Geometry: final body of the model. Coordinates: model frame, mm. A direction names the side the tool comes from. Give positions to 0.01 mm unless a question says otherwise; leave off trailing zeros. Loops run counter-clockwise (first coordinate to the right, second up) from the corner with the lowest first, then second, coordinate; pieces in that order, holes last.
1. First-contact query: P1, Ø1.4, axis at x = 63.5, z = 3, coming from the -Y side; P2, Ø1.1, axis at x = 71.5, z = 4.5, coming from the -Y side; P3, Ø3, axis at y = 36.5, z = 3, coming from the +X side; P4, Ø2, axis at x = 76.17, y = 8.42, coming from the +Z side. Flat tips, straight axial feed; report the tip coordinate or a pass-through.
2. Section A-A, the plane y = 15. Output: boundary loops of the cut face in (x, z).
3. Section D-D, the plane z = 8. State how many separate pieces and enclosed holes the cut face has, then the cut area to 3 significant figures.
4. Access query for faces 5 (the face through (71.515, 21.67, 6.958)), 6 (the face through (8, 45.25, 5)), 7 (the face through (18.611, 28, 2)). Directions: +Z, -Z, +X, -X, +Y, -Y. A direction counts if a zero-diameter tool reaches every point of the face in a straight line with its end or side. Return the directions, or none.
5. Section C-C, the plane x = 15.5. Output: boundary loops of the cut face in (y, z).
6. Material intervals for line 1 along Y through (x, z) = (76, 8.5); line 2 along X through (y, z) = (28.5, 2); line 3 along Y through (x, z) = (38.5, 2.25), sorted ascending.
7. Section B-B, the plane x = 67.5. Output: boundary loops of the cut face in (y, z), then the cut area to 3 significant figures.
8. Draft query along Y for faces 1 (the face through (75, 55, 0)), 2 (the face through (25, 30.686, 2)), 3 (the face through (8, 34.334, 5)), 4 (the face through (31, 23.353, 7)). Return one class per face: +Y half, -Y half, draft (parallel to the pull), parting line (faces both ways), or undercut.
from build123d import *

# Parameters (mm, degrees)
SKETCH_1_W           = 85
SKETCH_1_H           = 65
EXTRUDE_1_DEPTH      = 10
CUT_EXTRUDE_1_REACH  = 109.471
SKETCH_2_R           = 1.7
CUT_EXTRUDE_2_REACH  = 109.471
SKETCH_3_W           = 85
SKETCH_3_H           = 65
CUT_EXTRUDE_4_REACH  = 102.464
CUT_EXTRUDE_7_DEPTH  = 6
CUT_EXTRUDE_8_DEPTH  = 6
CUT_EXTRUDE_11_DEPTH = 4
SKETCH_8_W           = 8
SKETCH_8_H           = 5
CUT_EXTRUDE_12_DEPTH = 1
SKETCH_10_W          = 5.4
SKETCH_10_H          = 6
SKETCH_10_W_2        = 4
EXTRUDE_2_DEPTH      = 3.04
SKETCH_11_W          = 4.2
SKETCH_11_H          = 5
EXTRUDE_3_DEPTH      = 2.300115
SKETCH_12_W          = 12
SKETCH_12_H          = 6
EXTRUDE_4_DEPTH      = 2.89
SKETCH_13_W          = 6.499986347
SKETCH_13_H          = 5.115524378
EXTRUDE_5_DEPTH      = 3.6
SKETCH_14_W          = 6
SKETCH_14_H          = 7
EXTRUDE_6_DEPTH      = 2.890002
SKETCH_15_W          = 14
SKETCH_15_H          = 4.4
CUT_EXTRUDE_13_DEPTH = 6
CHAMFER_1_SIZE       = 1
CHAMFER_2_SIZE       = 0.6
CHAMFER_3_SIZE       = 0.6
CHAMFER_4_SIZE       = 0.6
CHAMFER_5_SIZE       = 0.6
CHAMFER_6_SIZE       = 0.6


with BuildPart() as part:
    # 草图1 → 凸台-拉伸1 (new body)
    with BuildSketch(Plane.XY):
        with Locations((42.5, 32.5)):
            Rectangle(SKETCH_1_W, SKETCH_1_H)
    extrude(amount=EXTRUDE_1_DEPTH)

    # 草图2 → 切除-拉伸1 (cut, up to next)
    with BuildSketch(Plane(origin=(0, 0, 0), x_dir=(-1, 0, 0), z_dir=(0, 0, -1)), mode=Mode.PRIVATE) as cut_extrude_1_sk1:
        with Locations((-76.166921514, 56.442524765)):
            Circle(SKETCH_2_R)
    cut_extrude_1_tool1 = extrude(cut_extrude_1_sk1.sketch, amount=-CUT_EXTRUDE_1_REACH, mode=Mode.PRIVATE) & part.part
    # 草图2 → 切除-拉伸1 (cut, up to next)
    with BuildSketch(Plane(origin=(0, 0, 0), x_dir=(-1, 0, 0), z_dir=(0, 0, -1)), mode=Mode.PRIVATE) as cut_extrude_1_sk2:
        with Locations((-8.888803658, 56.442524765)):
            Circle(SKETCH_2_R)
    cut_extrude_1_tool2 = extrude(cut_extrude_1_sk2.sketch, amount=-CUT_EXTRUDE_1_REACH, mode=Mode.PRIVATE) & part.part
    # 草图2 → 切除-拉伸1 (cut, up to next)
    with BuildSketch(Plane(origin=(0, 0, 0), x_dir=(-1, 0, 0), z_dir=(0, 0, -1)), mode=Mode.PRIVATE) as cut_extrude_1_sk3:
        with Locations((-76.166921514, 8.41508509)):
            Circle(SKETCH_2_R)
    cut_extrude_1_tool3 = extrude(cut_extrude_1_sk3.sketch, amount=-CUT_EXTRUDE_1_REACH, mode=Mode.PRIVATE) & part.part
    # 草图2 → 切除-拉伸1 (cut, up to next)
    with BuildSketch(Plane(origin=(0, 0, 0), x_dir=(-1, 0, 0), z_dir=(0, 0, -1)), mode=Mode.PRIVATE) as cut_extrude_1_sk4:
        with Locations((-8.888803658, 8.41508509)):
            Circle(SKETCH_2_R)
    cut_extrude_1_tool4 = extrude(cut_extrude_1_sk4.sketch, amount=-CUT_EXTRUDE_1_REACH, mode=Mode.PRIVATE) & part.part
    add(cut_extrude_1_tool1.solids().sort_by_distance((76.166922, 56.442525, 0))[0], mode=Mode.SUBTRACT)
    add(cut_extrude_1_tool2.solids().sort_by_distance((8.888804, 56.442525, 0))[0], mode=Mode.SUBTRACT)
    add(cut_extrude_1_tool3.solids().sort_by_distance((76.166922, 8.415085, 0))[0], mode=Mode.SUBTRACT)
    add(cut_extrude_1_tool4.solids().sort_by_distance((8.888804, 8.415085, 0))[0], mode=Mode.SUBTRACT)

    # 草图3 → 切除-拉伸2 (cut, up to next)
    with BuildSketch(Plane(origin=(0, 0, 0), x_dir=(-1, 0, 0), z_dir=(0, 0, -1)), mode=Mode.PRIVATE) as cut_extrude_2_sk1:
        with Locations((-42.5, 32.5)):
            Rectangle(SKETCH_3_W, SKETCH_3_H)
        Polygon((-5, 33.462892894), (-5.871324699, 34.334217592), (-5.87504445, 53.137061214), (-5, 54.017366187), (-5, 57.982143592), (-6.992565577, 59.974709169), (-23.773560915, 59.974709169), (-24.394872914, 59.353397171), (-54.61482093, 59.349677419), (-55.245113202, 59.974709169), (-77.982184232, 59.974709169), (-79.974749809, 57.982143592), (-79.97474981, 54.295829484), (-78.032030648, 52.353110322), (-78.028310897, 12.45999492), (-79.97474981, 10.508295484), (-79.97474981, 6.992565577), (-77.982184232, 5), (-74.414239441, 5), (-73.152434681, 6.26180476), (-60.043505207, 6.265524511), (-58.772720173, 5), (-32.926479725, 5), (-31.743585303, 6.182894422), (-17.461559563, 6.186614173), (-16.269684867, 5), (-6.992565577, 5), (-5, 6.992565577), align=None, mode=Mode.SUBTRACT)
    cut_extrude_2_tool1 = extrude(cut_extrude_2_sk1.sketch, amount=-CUT_EXTRUDE_2_REACH, mode=Mode.PRIVATE) & part.part
    add(cut_extrude_2_tool1.solids().sort_by_distance((42.5, 63.929953, 0))[0], mode=Mode.SUBTRACT)

    # 草图4 → 切除-拉伸4 (cut, up to next)
    with BuildSketch(Plane(origin=(0, 0, 0), x_dir=(-1, 0, 0), z_dir=(0, 0, -1)), mode=Mode.PRIVATE) as cut_extrude_4_sk1:
        Polygon((-73.152434681, 6.26180476), (-73.152434681, 20.032317315), (-69.831576581, 23.353175415), (-46.787984184, 23.353175415), (-20.851296271, 23.353175415), (-17.461559563, 19.963438707), (-17.461559563, 6.186614173), (-17.461559563, 0.193960815), (-73.152434681, 0.193960815), align=None)
    cut_extrude_4_tool1 = extrude(cut_extrude_4_sk1.sketch, amount=-CUT_EXTRUDE_4_REACH, mode=Mode.PRIVATE) & part.part
    add(cut_extrude_4_tool1.solids().sort_by_distance((45.311727, 11.681443, 0))[0], mode=Mode.SUBTRACT)

    # 草图5 → 切除-拉伸7 (cut)
    with BuildSketch(Plane(origin=(0, 0, 0), x_dir=(-1, 0, 0), z_dir=(0, 0, -1))):
        Polygon((-24.394872914, 59.353397171), (-24.394872914, 53.906418167), (-25.526104495, 52.774908066), (-53.482640788, 52.774908066), (-54.614150889, 53.906139647), (-54.61482093, 59.349677419), align=None)
    extrude(amount=-CUT_EXTRUDE_7_DEPTH, mode=Mode.SUBTRACT)

    # 草图6 → 切除-拉伸8 (cut)
    with BuildSketch(Plane(origin=(0, 0, 0), x_dir=(-1, 0, 0), z_dir=(0, 0, -1))):
        Polygon((-5.871324699, 34.334217592), (-11.136213102, 34.334217592), (-11.687697798, 35.836171197), (-11.687697798, 43.836171197), (-10.273484235, 45.250384759), (-5.873484235, 45.250384759), align=None)
    extrude(amount=-CUT_EXTRUDE_8_DEPTH, mode=Mode.SUBTRACT)

    # 草图7 → 切除-拉伸11 (cut)
    with BuildSketch(Plane(origin=(0, 0, 0), x_dir=(-1, 0, 0), z_dir=(0, 0, -1))):
        Polygon((-74.432117646, 51.26230094), (-76.432117646, 51.26230094), (-78.031928938, 51.26230094), (-78.029847328, 28.93771831), (-75.029847328, 28.93771831), (-75.029847328, 13.93771831), (-73.152434681, 12.060305663), (-73.152434681, 20.032317315), (-69.831576581, 23.353175415), (-20.851296271, 23.353175415), (-17.461559563, 19.963438707), (-17.461559563, 6.186614173), (-16.269684867, 5), (-12.014024847, 5), (-12.014024847, 10.599811284), (-10.599811284, 12.014024847), (-6.599811284, 12.014024847), (-5, 12.014024847), (-5, 33.462892894), (-5.871324699, 34.334217592), (-11.136213102, 34.334217592), (-11.687697798, 35.836171197), (-11.687697798, 43.836171197), (-10.273484235, 45.250384759), (-5.873484235, 45.250384759), (-5.87504445, 53.137061214), (-9.87504445, 53.137061214), (-12.071959353, 55.333976117), (-12.071959353, 58.333976117), (-23.061659554, 58.333976117), (-23.732127818, 57.663342778), (-24.394872914, 57.663261201), (-24.394872914, 53.906418167), (-25.526104495, 52.774908066), (-53.482640788, 52.774908066), (-54.614150889, 53.906139647), (-54.61482093, 59.349677419), (-55.245113202, 59.974709169), (-71.319520701, 59.974709169), (-71.319520701, 58.374897885), (-71.319520701, 54.374897885), align=None)
    extrude(amount=-CUT_EXTRUDE_11_DEPTH, mode=Mode.SUBTRACT)

    # 草图8 → 切除-拉伸12 (cut)
    with BuildSketch(Plane(origin=(0, 0, 4), x_dir=(-1, 0, 0), z_dir=(0, 0, -1))):
        with Locations((-69.348077333, 43.45871309)):
            Rectangle(SKETCH_8_W, SKETCH_8_H)
    extrude(amount=-CUT_EXTRUDE_12_DEPTH, mode=Mode.SUBTRACT)

    # 草图10 → 凸台-拉伸2 (add)
    with BuildSketch(Plane(origin=(0, 0, 4), x_dir=(-1, 0, 0), z_dir=(0, 0, -1))):
        with Locations((-44.246532103, 31.889800214)):
            Rectangle(SKETCH_10_W, SKETCH_10_H)
        with Locations((-39.546532103, 31.889800214)):
            Rectangle(SKETCH_10_W_2, SKETCH_10_H)
        with Locations((-34.846532103, 31.889800214)):
            Rectangle(SKETCH_10_W, SKETCH_10_H)
    extrude(amount=EXTRUDE_2_DEPTH)

    # 草图11 → 凸台-拉伸3 (add)
    with BuildSketch(Plane(origin=(0, 0, 4), x_dir=(-1, 0, 0), z_dir=(0, 0, -1))):
        with Locations((-38.731800654, 41.192864876)):
            Rectangle(SKETCH_11_W, SKETCH_11_H)
    extrude(amount=EXTRUDE_3_DEPTH)

    # 草图12 → 凸台-拉伸4 (add)
    with BuildSketch(Plane(origin=(0, 0, 4), x_dir=(-1, 0, 0), z_dir=(0, 0, -1))):
        with Locations((-24.610605003, 27.685920752)):
            Rectangle(SKETCH_12_W, SKETCH_12_H)
    extrude(amount=EXTRUDE_4_DEPTH)

    # 草图13 → 凸台-拉伸5 (add)
    with BuildSketch(Plane(origin=(0, 0, 4), x_dir=(-1, 0, 0), z_dir=(0, 0, -1))):
        with Locations((-61.319842519, 38.061085021)):
            Rectangle(SKETCH_13_W, SKETCH_13_H)
    extrude(amount=EXTRUDE_5_DEPTH)

    # 草图14 → 凸台-拉伸6 (add)
    with BuildSketch(Plane(origin=(0, 0, 4), x_dir=(-1, 0, 0), z_dir=(0, 0, -1))):
        with Locations((-62.740849727, 27.111901224)):
            Rectangle(SKETCH_14_W, SKETCH_14_H)
    extrude(amount=EXTRUDE_6_DEPTH)

    # 草图15 → 切除-拉伸13 (cut)
    with BuildSketch(Plane.XY.offset(10)):
        with Locations((48.428848604, 25.553175415)):
            Rectangle(SKETCH_15_W, SKETCH_15_H)
    extrude(amount=-CUT_EXTRUDE_13_DEPTH, mode=Mode.SUBTRACT)

    # 倒角1
    chamfer_1_edges = [part.edges().sort_by_distance(p)[0] for p in [
        (55.428848604, 23.353175415, 7),
        (55.428848604, 27.753175415, 7),
        (41.428848604, 27.753175415, 7),
        (41.428848604, 23.353175415, 7),
    ]]
    chamfer(chamfer_1_edges, length=CHAMFER_1_SIZE)

    # 倒角2
    chamfer_2_edges = [part.edges().sort_by_distance(p)[0] for p in [
        (64.569835693, 38.061085021, 4),
        (61.31984252, 35.503322832, 4),
        (58.069849346, 38.061085021, 4),
        (61.31984252, 40.61884721, 4),
    ]]
    chamfer(chamfer_2_edges, length=CHAMFER_2_SIZE)

    # 倒角3
    chamfer_3_edges = [part.edges().sort_by_distance(p)[0] for p in [
        (39.546532103, 28.889800214, 4),
        (46.946532103, 31.889800214, 4),
        (39.546532103, 34.889800214, 4),
        (32.146532103, 31.889800214, 4),
    ]]
    chamfer(chamfer_3_edges, length=CHAMFER_3_SIZE)

    # 倒角4
    chamfer_4_edges = [part.edges().sort_by_distance(p)[0] for p in [
        (30.610605003, 27.685920752, 4),
        (24.610605003, 24.685920752, 4),
        (18.610605003, 27.685920752, 4),
        (24.610605003, 30.685920752, 4),
    ]]
    chamfer(chamfer_4_edges, length=CHAMFER_4_SIZE)

    # 倒角5
    chamfer_5_edges = [part.edges().sort_by_distance(p)[0] for p in [
        (40.831800654, 41.192864876, 4),
        (38.731800654, 38.692864876, 4),
        (36.631800654, 41.192864876, 4),
        (38.731800654, 43.692864876, 4),
    ]]
    chamfer(chamfer_5_edges, length=CHAMFER_5_SIZE)

    # 倒角6
    chamfer_6_edges = [part.edges().sort_by_distance(p)[0] for p in [
        (65.740849727, 27.111901224, 4),
        (59.740849727, 27.111901224, 4),
        (62.740849727, 30.611901224, 4),
    ]]
    chamfer(chamfer_6_edges, length=CHAMFER_6_SIZE)


solid = part.part
Answers below:
1. P1: stops at y = 23.61
1. P2: stops at y = 21.13
1. P3: stops at x = 78.03
1. P4: passes through
2. outline: (5, 4) - (17.46, 4) - (17.46, 10) - (5, 10) - close; (73.15, 4) - (75.03, 4) - (75.03, 0) - (78.03, 0) - (78.03, 10) - (73.15, 10) - close
3. separate pieces: 1
3. enclosed holes: 4
3. area: 2,890 mm2
4. face 5: +Z, -Z, -Y
4. face 6: -Z, -X
4. face 7: -Z, -X, -Y
5. outline: (5, 4) - (58.33, 4) - (58.33, 0) - (59.97, 0) - (59.97, 10) - (5, 10) - close
6. line 1: y = 5 to 6.72, 10.11 to 54.75, 58.13 to 59.97
6. line 2: x = 18.61 to 30.61, 59.74 to 65.74, 75.03 to 78.03
6. line 3: y = 28.89 to 34.89, 38.69 to 43.69
7. outline: (23.35, 4) - (40.96, 4) - (40.96, 5) - (45.96, 5) - (45.96, 4) - (59.97, 4) - (59.97, 10) - (23.35, 10) - close
7. area: 215 mm2
8. face 1: draft
8. face 2: undercut
8. face 3: undercut
8. face 4: -Y half
